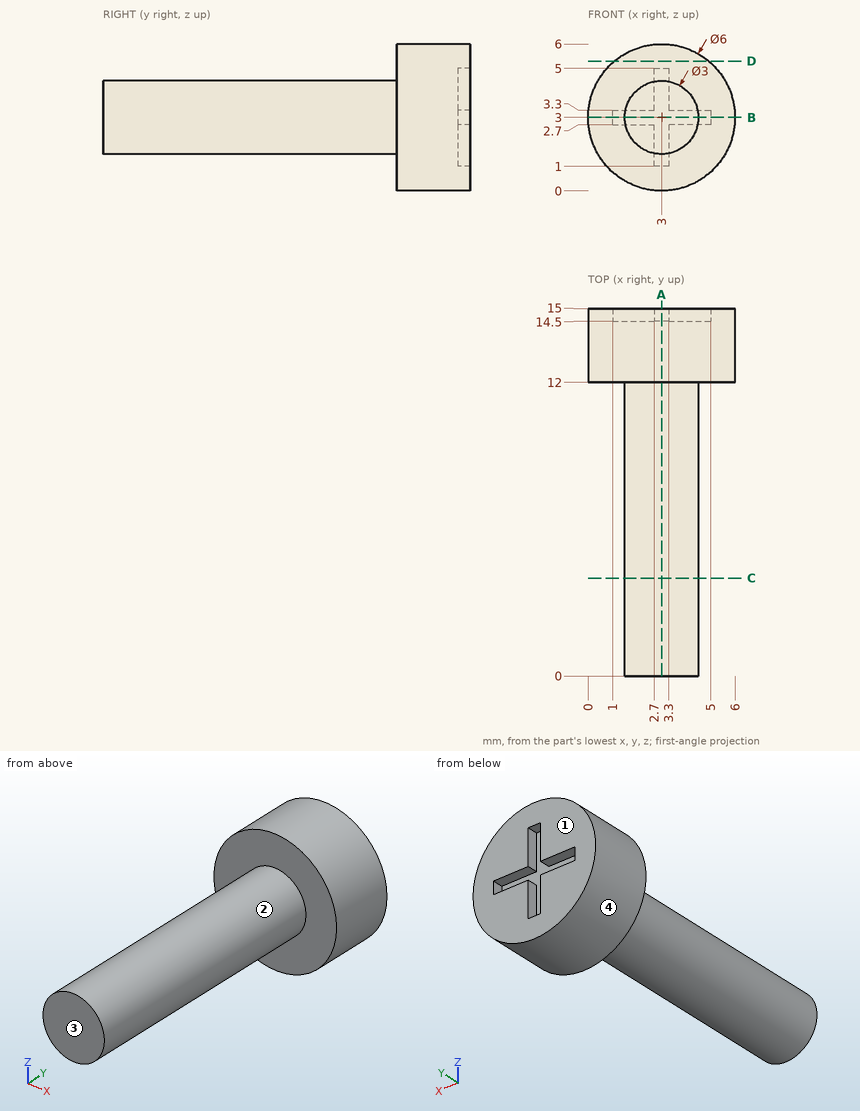
Geometry check sheet. Reference: drawing and pictorial views, mm from the part's lowest x, y, z. A direction names the side the tool comes from. Coordinates: 2 decimals unless noted, no trailing zeros. Write each loop counter-clockwise with the first axis right and the second up, starting at its lowest first coordinate (ties: lowest second). Pieces come first, ordered by that corner, then holes. Notation, with made-up numbers: (-25.5, 20.25) - (25.5, 20.25) arc R25 cw to (25.5, 52.25) - close; hole circle Ø10 at (-24, 74). An arc over 180 degrees is marked (long way). One line per question, with ' | ' between items. Start each with the question number.
1. Access from +Z, -Z, +X, -X, +Y, -Y to the whole of each face (thin tool, end or side, straight path). Record for the marked faces 1 and 2.
2. Gauge pin test, flat ends, axial feed: P1, Ø0.6, axis at y = 14.5, z = 1.5, coming from the +X side; P2, Ø0.6, axis at x = 4, y = 14.5, coming from the +Z side; P3, Ø3, axis at y = 3.5, z = 1.5, coming from the +X side. Record the tip position at first contact, or that the pin passes through.
3. Material ranges on line 1 along Y through (x, z) = (4.85, 1.05); line 2 along Y through (x, z) = (1.65, 2.8); line 3 along X through (y, z) = (14, 3.15), recorded low to high.
4. Section check B-B (z = 3). Enter the section's corners in (x, y).
5. Section check A-A (x = 3). Enter the section's corners in (y, z).
6. Section check D-D (z = 5.3). Enter the section's corners in (x, y), plus the area to 3 significant figures.
7. Section check C-C (y = 4). Enter the section's corners in (x, z).
8. Draft check along X on the marked faces 3 and 4. Enter one of: released by +X, released by -X, zero draft, split by the parting line, or undercut.
Computed values:
1) face 1: +Z, -Z, +X, -X, +Y | face 2: -Y
2) P1: x = 5.75 | P2: z = 5.92 | P3: x = 4.5
3) line 1: 12 to 15 | line 2: 0 to 14.5 | line 3: 0 to 6
4) outline: (0, 12) - (1.5, 12) - (1.5, 0) - (4.5, 0) - (4.5, 12) - (6, 12) - (6, 15) - (5, 15) - (5, 14.5) - (1, 14.5) - (1, 15) - (0, 15) - close
5) outline: (0, 1.5) - (12, 1.5) - (12, 0) - (15, 0) - (15, 1) - (14.5, 1) - (14.5, 5) - (15, 5) - (15, 6) - (12, 6) - (12, 4.5) - (0, 4.5) - close
6) outline: (1.07, 12) - (4.93, 12) - (4.93, 15) - (1.07, 15) - close | area: 11.6 mm²
7) outline: circle Ø3 at (3, 3)
8) face 3: zero draft | face 4: split by the parting line
